Model file for the job. Use its own axes, mm. A direction names the side the tool comes from. Coordinates: 2 decimals unless noted, no trailing zeros. Order: outer loops, then holes, each group sorted by start corner. A loop starts at its lowest first (then second) coordinate and runs counter-clockwise, first axis right, second up. Notation, with made-up numbers: (-26, -24.5) -> (-3, -24.5) arc R28 ccw to (-3, -4.5) -> close; hole circle Ø2 at (86, 10.5). An arc over 180 degrees is marked (long way). Write item = value, one per line. Start each with the question number.
Q1. Cut at C-C, the plane y = 11. Give the number of separate pieces and of enclosed holes in the cut face, plus the area to 3 significant figures.
Q2. Cut at A-A, the plane x = 0. List the corners of the cut face in (y, z), plus the area to 3 significant figures.
Q3. Wall check: line 1 (Z direction, x = 31, y = 19.5); line 2 (Y direction, x = 0, z = 23); line 3 (Y direction, x = 25, z = -20.5). Give the ranges that are in metal, low to high. Write a range as from..to.
Q4. Flat gauge pins, fed straight in: pin 1 (3 mm diameter, centred on x = -19, z = -7, fed in from +Y); pin 2 (3 mm diameter, centred on x = -25, y = 12, fed in from +Z); pin 3 (3 mm diameter, centred on y = 5.5, z = 7, fed in from +X); pin 4 (6 mm diameter, centred on x = -15.5, z = 16.5, fed in from +Y). Where does each tip first touch, or does it go through?
Q5. Cut at B-B, the plane z = -10.5. List the corners of the cut face in (x, y).
Q6. Mould opens along Z. For faces 1 (the face through (24.46, 9.56, -20.49)), 2 (the face through (23.25, 12.08, -22.97)), 3 (the face through (0, 14, -25)) say: +Z half, -Z half, draft (parallel to the pull), parting line (faces both ways), or undercut.
Q7. 3-axis set-ups, long thin cutter, end or side, ignore diameter. For faces 4 (the face through (-34.43, 10.48, 20.6)), 5 (the face through (-2, 19, -21)), 6 (the face through (0.51, 11.74, 0.31)), 7 (the face through (34.825, 19.652, 23.045)): which of +Z, -Z, +X, -X, +Y, -Y reach the whole face in a straight line?
from build123d import *

# Parameters (mm, degrees)
PAD001_DEPTH    = 25
POCKET_DEPTH    = 20
FILLET_R        = 2
SKETCH002_R     = 1.75
POCKET001_DEPTH = 50.001
SKETCH003_R     = 2.5
POCKET002_DEPTH = 1


with BuildPart() as part:
    # Sketch001 → Pad001 (new body, symmetric)
    with BuildSketch(Plane.XY):
        with BuildLine():
            Line((-35, 20), (-35, 0))
            Line((-35, 0), (35, 0))
            Line((35, 0), (35, 20))
            ThreePointArc((35, 20), (0, 29.378222), (-35, 20))
        make_face()
    extrude(amount=PAD001_DEPTH, both=True)

    # Sketch → Pocket (cut, symmetric)
    with BuildSketch(Plane.XY):
        with BuildLine():
            ThreePointArc((37.264344, 1), (0, 11.743197), (-37.264344, 1))
            Line((-37.264344, 1), (-37.264344, 41.61153))
            Line((-37.264344, 41.61153), (37.264344, 41.61153))
            Line((37.264344, 41.61153), (37.264344, 1))
        make_face()
    extrude(amount=POCKET_DEPTH, both=True, mode=Mode.SUBTRACT)

    # Fillet
    fillet_edges = [part.edges().sort_by_distance(p)[0] for p in [
        (0, 29.378222, 25),
        (-35, 20, 22.5),
        (0, 29.378222, 20),
        (0, 29.378222, -20),
        (-35, 20, -22.5),
        (0, 29.378222, -25),
        (35, 20, 22.5),
        (35, 20, -22.5),
        (35, 11.182488, -20),
        (35, 11.182488, 20),
        (-35, 11.182488, -20),
        (-35, 11.182488, 20),
    ]]
    fillet(fillet_edges, radius=FILLET_R)

    # Sketch002 (on DatumPlane) → Pocket001 (cut, through all)
    with BuildSketch(Plane.XY.offset(25)):
        with Locations((0, 20)):
            Circle(SKETCH002_R)
        with Locations((25, 12)):
            Circle(SKETCH002_R)
        with Locations((-25, 12)):
            Circle(SKETCH002_R)
    extrude(amount=-POCKET001_DEPTH, mode=Mode.SUBTRACT)

    # Sketch003 (on DatumPlane) → Pocket002 (cut)
    with BuildSketch(Plane.XY.offset(-20)):
        with Locations((0, 20)):
            Circle(SKETCH003_R)
        with Locations((-25, 12)):
            Circle(SKETCH003_R)
        with Locations((25, 12)):
            Circle(SKETCH003_R)
    extrude(amount=-POCKET002_DEPTH, mode=Mode.SUBTRACT)


solid = part.part
Here are the results:
q1.separate_pieces = 5
q1.enclosed_holes = 0
q1.area = 1,450 mm²
q2.outline = (0, -25) -> (18.25, -25) -> (18.25, -21) -> (17.5, -21) -> (17.5, -20) -> (11.74, -20) -> (11.74, 20) -> (18.25, 20) -> (18.25, 25) -> (0, 25) -> close; (21.75, -25) -> (27.38, -25) arc R2 ccw to (29.38, -23) -> (29.38, -22) arc R2 ccw to (27.38, -20) -> (22.5, -20) -> (22.5, -21) -> (21.75, -21) -> close; (21.75, 20) -> (27.38, 20) arc R2 ccw to (29.38, 22) -> (29.38, 23) arc R2 ccw to (27.38, 25) -> (21.75, 25) -> close
q2.area = 724 mm²
q3.line_1 = -25..-20, 20..25
q3.line_2 = 0..18.25, 21.75..29.38
q3.line_3 = 0..9.5, 14.5..24.04
q4.pin_1 = 9.52
q4.pin_2 = through
q4.pin_3 = 32
q4.pin_4 = 10.62
q5.outline = (-35, 0) -> (35, 0) -> (35, 2.36) arc R70 ccw to (-35, 2.36) -> close
q6.face_1 = undercut
q6.face_2 = draft
q6.face_3 = -Z half
q7.face_4 = -X, +Y
q7.face_5 = none
q7.face_6 = +Y
q7.face_7 = +Z, -Z, +X, +Y
